Geometry: final body of the model. Coordinates: model frame, mm. Face numbers are marked on the shaded views. A direction names the side the tool comes from. Round coordinates to 2 decimals unless told otherwise and drop trailing zeros. Loops run counter-clockwise (first coordinate to the right, second up) from the corner with the lowest first, then second, coordinate; pieces in that order, holes last. Notation, with made-up numbers: (37, -13.75) -> (44, -13.75) arc R27 ccw to (44, 5.25) -> close; hole circle Ø7 at (-5, 20). An arc over 180 degrees is marked (long way). Answer in a Markdown table with one row per item.
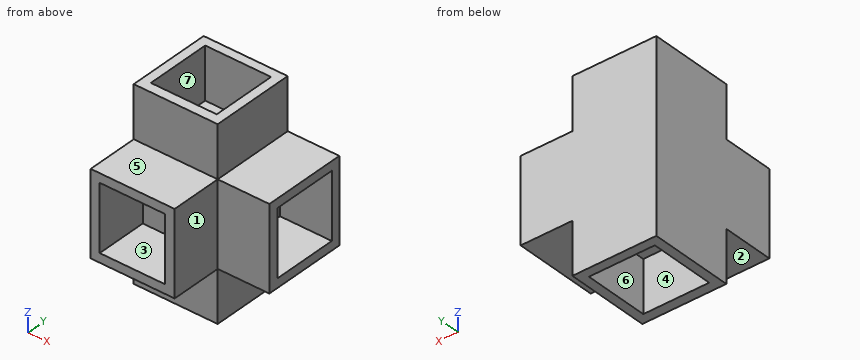
```python
from build123d import *

# Parameters (mm, degrees)
F0_W          = 13
F0_H          = 21
F1_DEPTH      = 13
F3_W          = 13
F3_H          = 13
F4_DEPTH      = 8
F4_DEPTH_BACK = 21
F5_W          = 10.2
F5_H          = 10.1
F6_DEPTH      = 8
F7_W          = 10.2
F7_H          = 10.1
F8_DEPTH      = 8
F9_W          = 13
F9_H          = 13
F10_DEPTH     = 8
F2_W          = 10.1
F2_H          = 10.2
F12_DEPTH     = 8
F11_W         = 10.1
F11_H         = 10.2
F13_DEPTH     = 8


with BuildPart() as f1:
    # F0 (on Top) → F1 (new body)
    with BuildSketch(Plane.XY):
        with Locations((-21.92968, -0.716216)):
            Rectangle(F0_W, F0_H)
    extrude(amount=F1_DEPTH)

    # F3 (on face) → F4 (join, two sides)
    with BuildSketch(Plane.XY.offset(13)) as f4_sk:
        with Locations((-21.92968, 3.283784)):
            Rectangle(F3_W, F3_H)
    extrude(amount=F4_DEPTH)
    extrude(f4_sk.sketch, amount=-F4_DEPTH_BACK)

    # F5 (on face) → F6 (cut)
    with BuildSketch(Plane.XY.offset(21)):
        with Locations((-21.92968, 3.333784)):
            Rectangle(F5_W, F5_H)
    extrude(amount=-F6_DEPTH, mode=Mode.SUBTRACT)

    # F7 (on face) → F8 (cut)
    with BuildSketch(Plane(origin=(0, 0, -8), x_dir=(1, 0, 0), z_dir=(0, 0, -1))):
        with Locations((-21.92968, -3.333784)):
            Rectangle(F7_W, F7_H)
    extrude(amount=-F8_DEPTH, mode=Mode.SUBTRACT)

    # F9 (on face) → F10 (join)
    with BuildSketch(Plane.YZ.offset(-15.42968)):
        with Locations((3.283784, 6.5)):
            Rectangle(F9_W, F9_H)
    extrude(amount=F10_DEPTH)

    # F2 (on face) → F12 (cut)
    with BuildSketch(Plane.XZ.offset(11.216216)):
        with Locations((-21.97968, 6.5)):
            Rectangle(F2_W, F2_H)
    extrude(amount=-F12_DEPTH, mode=Mode.SUBTRACT)

    # F11 (on face) → F13 (cut)
    with BuildSketch(Plane.YZ.offset(-7.42968)):
        with Locations((3.333784, 6.5)):
            Rectangle(F11_W, F11_H)
    extrude(amount=-F13_DEPTH, mode=Mode.SUBTRACT)


solid = f1.part
```
Item 1: Draft query along X for the marked faces 1, 2, 3 and 4. Return one class per face: pulls with the +X half, pulls with the -X half, needs draft (parallel to the pull), parting line crosses it, or undercut.
Answer:
| item | result |
|---|---|
| face 1 | pulls with the +X half |
| face 2 | needs draft |
| face 3 | undercut |
| face 4 | undercut |
Item 2: Cut plane D-D (y = 4.5). Output: boundary loops of the cut face in (x, z), then the cut area to 3 significant figures.
Answer:
| item | result |
|---|---|
| outline | (-28.43, -8) -> (-27.03, -8) -> (-27.03, 0) -> (-16.83, 0) -> (-16.83, -8) -> (-15.43, -8) -> (-15.43, 0) -> (-7.43, 0) -> (-7.43, 1.4) -> (-15.43, 1.4) -> (-15.43, 11.6) -> (-7.43, 11.6) -> (-7.43, 13) -> (-15.43, 13) -> (-15.43, 21) -> (-16.83, 21) -> (-16.83, 13) -> (-27.03, 13) -> (-27.03, 21) -> (-28.43, 21) -> close |
| area | 236 mm² |
Item 3: Cut plane C-C (z = 6). Output: boundary loops of the cut face in (x, y).
Answer:
| item | result |
|---|---|
| outline | (-28.43, -11.22) -> (-27.03, -11.22) -> (-27.03, -3.22) -> (-16.93, -3.22) -> (-16.93, -11.22) -> (-15.43, -11.22) -> (-15.43, -3.22) -> (-7.43, -3.22) -> (-7.43, -1.72) -> (-15.43, -1.72) -> (-15.43, 8.38) -> (-7.43, 8.38) -> (-7.43, 9.78) -> (-28.43, 9.78) -> close |
Item 4: Cut plane A-A (y = -9.5). Output: boundary loops of the cut face in (x, z), then the cut area to 3 significant figures.
Answer:
| item | result |
|---|---|
| outline | (-28.43, 0) -> (-15.43, 0) -> (-15.43, 13) -> (-28.43, 13) -> close; hole (-27.03, 1.4) -> (-16.93, 1.4) -> (-16.93, 11.6) -> (-27.03, 11.6) -> close |
| area | 66.0 mm² |
Item 5: Cut plane B-B (z = -1.75). Output: boundary loops of the cut face in (x, y), then the cut area to 3 significant figures.
Answer:
| item | result |
|---|---|
| outline | (-28.43, -3.22) -> (-15.43, -3.22) -> (-15.43, 9.78) -> (-28.43, 9.78) -> close; hole (-27.03, -1.72) -> (-16.83, -1.72) -> (-16.83, 8.38) -> (-27.03, 8.38) -> close |
| area | 66.0 mm² |
Item 6: Reachability of the marked faces 5, 6 and 7 from +Z, -Z, +X, -X, +Y, -Y: full face, straight path, thin tool, end or side. Return the list, or none.
Answer:
| item | result |
|---|---|
| face 5 | +Z, +X, -X, -Y |
| face 6 | -Z |
| face 7 | +Z |
Item 7: Line query: probe 1 along X at (y, z) = (1, -6); probe 2 along Y at (x, z) = (-26.5, 16.25); probe 3 along X at (y, z) = (-0.75, 5.25). Output: solid intervals per line, ascending. Write a range as [from, to].
Answer:
| item | result |
|---|---|
| probe 1 | x = [-28.43, -27.03], [-16.83, -15.43] |
| probe 2 | y = [-3.22, -1.72], [8.38, 9.78] |
| probe 3 | x = [-28.43, -15.43] |
Item 8: Pin query (flat end, axial travel): pin 1 Ø9 at (x, z) = (-11.5, 6.5) entering from -Y; pin 2 Ø3 at (x, y) = (-12, 5) entering from -Z; pin 3 Ø4 at (x, z) = (-23, -4) entering from -Y; pin 4 Ø4 at (y, z) = (-8.5, 8.5) entering from +X. Return the tip coordinate at first contact, or that it passes through.
Answer:
| item | result |
|---|---|
| pin 1 | stops at y = -11.22 |
| pin 2 | stops at z = 0 |
| pin 3 | stops at y = -3.22 |
| pin 4 | stops at x = -15.43 |
